Can you work these out from the model? Positions are in its coordinate system, mm. Coordinates: 2 decimals unless noted, no trailing zeros. Order: outer loops, then holes, each group sorted by start corner. A loop starts at its lowest first (then second) coordinate and runs counter-clockwise, first axis right, second up. Notation, with made-up numbers: (-17.75, -27) -> (21.25, -27) arc R32 cw to (21.25, 9) -> close; hole circle Ø1 at (10.25, -37.5). An arc over 180 degrees is marked (long way). Return JSON: item names as keys, results as strings. Group by question number.
1) If we section it at B-B, the plane z = 0: Please give me the cut outline in (x, y), then the cut area to 3 significant figures.
2) If we section it at C-C, the plane y = 2.45: State how many separate pieces and enclosed holes the cut face has, then the cut area to 3 significant figures.
3) If I drill on probe 1 along X at (y, z) = (4.2, 0.5); probe 2 along X at (y, z) = (1, 10.25); probe 3 along X at (y, z) = (2.85, -11), over which ranges is the centre line in solid material (lowest first)? Write a range as from..to.
4) If we section it at A-A, the plane x = 0: Please give me the cut outline in (y, z).
5) If we section it at D-D, the plane z = 9: Please give me the cut outline in (x, y), then the cut area to 3 significant figures.
6) Thinking about a two-plate mould opening in X: for faces 1 (the cylindrical face through (-0.413, 2.739, -8.528)), 2 (the cylindrical face through (5.4, 2.82, 11.79)), 3 (the cylindrical face through (0.047, 2.739, 8.447)), 4 (the flat face through (-3, 0, 0)), which applies, +X half, -X half, draft (parallel to the pull), parting line (faces both ways), or undercut?
from build123d import *

# Parameters (mm, degrees)
SKETCH1_W      = 15.65275
SKETCH1_H      = 25.4
SKETCH1_R      = 1.89865
SKETCH1_R_2    = 1.0795
EXTRUDE1_DEPTH = 5.55625
FILLET1_R      = 3.175


with BuildPart() as part:
    # Sketch1 → Extrude1 (new body)
    with BuildSketch(Plane(origin=(0, 0, 0), x_dir=(1, 0, 0), z_dir=(0, 1, 0))):
        with Locations((-1.476375, 0)):
            Rectangle(SKETCH1_W, SKETCH1_H)
        with Locations(Location((0, 0, 0), (0, 0, 270))):
            Circle(SKETCH1_R, mode=Mode.SUBTRACT)
        with Locations(Location((0, 9.525, 0), (0, 0, 270))):
            Circle(SKETCH1_R_2, mode=Mode.SUBTRACT)
        with Locations(Location((0, -9.525, 0), (0, 0, 270))):
            Circle(SKETCH1_R_2, mode=Mode.SUBTRACT)
    extrude(amount=EXTRUDE1_DEPTH)

    # Fillet1
    fillet1_edges = [part.edges().sort_by_distance(p)[0] for p in [
        (6.35, 2.778125, -12.7),
        (6.35, 2.778125, 12.7),
    ]]
    fillet(fillet1_edges, radius=FILLET1_R)


solid = part.part
Result sheet:
{
 "1": {"outline": "(-9.3, 0) -> (-1.9, 0) -> (-1.9, 5.56) -> (-9.3, 5.56) -> close; (1.9, 0) -> (6.35, 0) -> (6.35, 5.56) -> (1.9, 5.56) -> close", "area": "65.9 mm2"},
 "2": {"separate pieces": "1", "enclosed holes": "3", "area": "375 mm2"},
 "3": {"probe 1": "x = -9.3..-1.83, 1.83..6.35", "probe 2": "x = -9.3..-0.8, 0.8..6.27", "probe 3": "x = -9.3..5.99"},
 "4": {"outline": "(0, -12.7) -> (5.56, -12.7) -> (5.56, -10.6) -> (0, -10.6) -> close; (0, -8.45) -> (5.56, -8.45) -> (5.56, -1.9) -> (0, -1.9) -> close; (0, 1.9) -> (5.56, 1.9) -> (5.56, 8.45) -> (0, 8.45) -> close; (0, 10.6) -> (5.56, 10.6) -> (5.56, 12.7) -> (0, 12.7) -> close"},
 "5": {"outline": "(-9.3, 0) -> (-0.94, 0) -> (-0.94, 5.56) -> (-9.3, 5.56) -> close; (0.94, 0) -> (6.35, 0) -> (6.35, 5.56) -> (0.94, 5.56) -> close", "area": "76.5 mm2"},
 "6": {"face 1": "undercut", "face 2": "+X half", "face 3": "undercut", "face 4": "draft"}
}
